```python
from build123d import *

# Parameters (mm, degrees)
SKETCH1_R           = 2.38125
SKETCH1_R_2         = 2.1828125
BOSS_EXTRUDE1_DEPTH = 6.35
CHAMFER1_SIZE       = 3.175
CHAMFER2_SIZE       = 0.396875


with BuildPart() as part:
    # Sketch1 → Boss-Extrude1 (new body)
    with BuildSketch(Plane(origin=(0, 0, 0), x_dir=(1, 0, 0), z_dir=(0, 1, 0))):
        Polygon((-44.45, 6.35), (62.365403734, 6.35), (119.934787808, -51.219384074), (110.954531687, -60.199640195), (57.104891492, -6.35), (-44.45, -6.35), align=None)
        with Locations(Location((-38.1, 0, 0), (0, 0, 270))):
            Circle(SKETCH1_R, mode=Mode.SUBTRACT)
        with Locations(Location((0, 0, 0), (0, 0, 270))):
            Circle(SKETCH1_R, mode=Mode.SUBTRACT)
        with Locations(Location((110.954531687, -51.219384074, 0), (0, 0, 270))):
            Circle(SKETCH1_R_2, mode=Mode.SUBTRACT)
        with Locations(Location((101.974275566, -42.239127953, 0), (0, 0, 270))):
            Circle(SKETCH1_R_2, mode=Mode.SUBTRACT)
        with Locations(Location((-12.7, 0, 0), (0, 0, 270))):
            Circle(SKETCH1_R_2, mode=Mode.SUBTRACT)
        with Locations(Location((25.4, 0, 0), (0, 0, 270))):
            Circle(SKETCH1_R_2, mode=Mode.SUBTRACT)
        with Locations(Location((84.013763324, -24.27861571, 0), (0, 0, 270))):
            Circle(SKETCH1_R_2, mode=Mode.SUBTRACT)
    extrude(amount=BOSS_EXTRUDE1_DEPTH)

    # Fillet1
    # the kernel refuses this chamfer: 50.8 mm, written as the material it adds along each edge
    with BuildSketch(Plane(origin=(57.104891492, 0, 6.35), x_dir=(0.7306772036716535, 0, 0.6827230946984092), z_dir=(0, 1, 0))) as fillet1_piece_1:
        with BuildLine():
            Line((22.93255988, 0), (-17.277556946, -15.079400804))
            Line((-17.277556946, -15.079400804), (-17.97120361, -14.337032765))
            ThreePointArc((-17.97120361, -14.337032765), (-9.066978051, -7.081424312), (-0.693646664, 0.742368039))
            Line((-0.693646664, 0.742368039), (0.034451214, 1.015415734))
            ThreePointArc((0.034451214, 1.015415734), (11.487547245, 0.626832956), (22.967011094, 1.015415734))
            Line((22.967011094, 1.015415734), (22.93255988, 0))
        make_face()
    extrude(amount=6.35)

    # Fillet2
    # the kernel refuses this chamfer: 57.15 mm, written as the material it takes off along each edge
    with BuildSketch(Plane(origin=(62.365403734, -64.497824661, -6.35), x_dir=(0.7306772036716533, 0, 0.6827230946984093), z_dir=(0, 1, 0))) as fillet2_piece_1:
        with BuildLine():
            Line((25.799129864, 0), (-19.437251564, -16.964325904))
            Line((-19.437251564, -16.964325904), (-20.217604061, -16.129161861))
            ThreePointArc((-20.217604061, -16.129161861), (-10.200350307, -7.966602351), (-0.780352497, 0.835164044))
            Line((-0.780352497, 0.835164044), (0.038757616, 1.142342701))
            ThreePointArc((0.038757616, 1.142342701), (12.923490651, 0.705187075), (25.837887481, 1.142342701))
            Line((25.837887481, 1.142342701), (25.799129864, 0))
        make_face()
    extrude(amount=135.345649322, mode=Mode.SUBTRACT)

    # Chamfer1
    chamfer1_edges = [part.edges().sort_by_distance(p)[0] for p in [
        (-44.45, 3.175, -6.35),
        (119.934787808, 3.175, 51.219384074),
        (110.954531687, 3.175, 60.199640195),
        (-44.45, 3.175, 6.35),
    ]]
    chamfer(chamfer1_edges, length=CHAMFER1_SIZE)

    # Chamfer2
    chamfer2_edges = [part.edges().sort_by_distance(p)[0] for p in [
        (0, 0, -2.38125),
        (0, 6.35, -2.38125),
        (-38.1, 0, -2.38125),
        (-38.1, 6.35, -2.38125),
        (110.954531687, 0, 49.036571574),
        (110.954531687, 6.35, 49.036571574),
        (101.974275566, 0, 40.056315453),
        (101.974275566, 6.35, 40.056315453),
        (-12.7, 0, -2.1828125),
        (-12.7, 6.35, -2.1828125),
        (25.4, 0, -2.1828125),
        (25.4, 6.35, -2.1828125),
        (84.013763324, 0, 22.09580321),
        (84.013763324, 6.35, 22.09580321),
        (90.346667332, 0, 39.59177584),
        (90.346667332, 6.35, 39.59177584),
        (54.023354766, 0, 13.789487758),
        (54.023354766, 6.35, 13.789487758),
        (-1.290950678, 0, -6.35),
        (-1.290950678, 6.35, -6.35),
        (58.898674917, 0, 2.019423728),
        (58.898674917, 6.35, 2.019423728),
        (-44.45, 0, 0),
        (-44.45, 6.35, 0),
        (98.396987484, 0, 29.681583749),
        (115.444659748, 0, 55.709512134),
        (-2.606078738, 0, 6.35),
        (117.689723778, 0, 51.219384074),
        (110.954531687, 0, 57.954576164),
        (-42.8625, 0, 4.7625),
        (-42.8625, 0, -4.7625),
        (98.396987484, 6.35, 29.681583749),
        (-2.606078738, 6.35, 6.35),
        (115.444659748, 6.35, 55.709512134),
        (117.689723778, 6.35, 51.219384074),
        (110.954531687, 6.35, 57.954576164),
        (-42.8625, 6.35, 4.7625),
        (-42.8625, 6.35, -4.7625),
    ]]
    chamfer(chamfer2_edges, length=CHAMFER2_SIZE)


solid = part.part
```
Source: CAD feature listing. Evaluate the final solid. Frame: model axes, mm. A direction names the side the tool comes from. Coordinates: 2 decimals unless noted, no trailing zeros. Write each loop counter-clockwise with the first axis right and the second up, starting at its lowest first coordinate (ties: lowest second). Pieces come first, ordered by that corner, then holes. Notation, with made-up numbers: (24.25, 2.25) - (64.25, 2.25) arc R17 cw to (64.25, 15.25) - close; hole circle Ø9 at (1, 37.5). An arc over 180 degrees is marked (long way). Answer as a JSON object with one key per item and string values.
Q1. Material intervals for line 1 (X direction, y = 4.4, z = 0); line 2 (X direction, y = 1.5, z = 49.5); line 3 (Z direction, x = -24, y = 4.25), sorted ascending. Write a range as [from, to].
Ans:
{"line 1": "x = [-44.45, -40.48], [-35.72, -14.88], [-10.52, -2.38], [2.38, 23.22], [27.58, 54.02]", "line 2": "x = [100.25, 109.61], [112.3, 117.69]", "line 3": "z = [-6.35, 6.35]"}
Q2. Section query B-B, the plane y = 2. State how many separate pieces and enclosed holes the cut face has, plus the area to 3 significant figures.
Ans:
{"separate pieces": "1", "enclosed holes": "7", "area": "2,150 mm2"}
Q3. First-contact query: pin 1 Ø3.5 at (x, z) = (84.01, 24.28) entering from -Y; pin 2 Ø1 at (x, y) = (83, 2.5) entering from +Z; pin 3 Ø3 at (x, y) = (-18, 4) entering from +Z; pin 4 Ø2 at (x, y) = (80, 5.5) entering from +Z. Flat tips, straight axial feed; report the tip coordinate or a pass-through.
Ans:
{"pin 1": "passes through", "pin 2": "stops at z = 32.75", "pin 3": "stops at z = 6.35", "pin 4": "stops at z = 30.25"}
Q4. Section query C-C, the plane x = -25. Output: boundary loops of the cut face in (y, z).
Ans:
{"outline": "(0, -5.95) - (0.4, -6.35) - (5.95, -6.35) - (6.35, -5.95) - (6.35, 5.95) - (5.95, 6.35) - (0.4, 6.35) - (0, 5.95) - close"}
Q5. Section query A-A, the plane x = 25.4. Output: boundary loops of the cut face in (y, z).
Ans:
{"outline": "(0, -5.95) - (0.4, -6.35) - (5.95, -6.35) - (6.35, -5.95) - (6.35, -2.58) - (5.95, -2.18) - (0.4, -2.18) - (0, -2.58) - close; (0, 2.58) - (0.4, 2.18) - (5.95, 2.18) - (6.35, 2.58) - (6.35, 5.95) - (5.95, 6.35) - (0.4, 6.35) - (0, 5.95) - close"}
Q6. Draft query along Z for faces 1 (the flat face through (115.334, 6.154, 55.536)), 2 (the cylindrical face through (23.463, 3.136, 1.007)), 3 (the flat face through (97.99, 0.2, 29.55)). Return one class per face: released by +Z, released by -Z, zero draft, split by the parting line, or undercut.
Ans:
{"face 1": "released by +Z", "face 2": "undercut", "face 3": "released by -Z"}
Q7. Set-up query: faces 4 (the flat face through (-2, 3, 6.35)), 5 (the flat face through (-42.7, 0.2, -4.65)). Return all of +Z, -Z, +X, -X, +Y, -Y with unobstructed straight access to the full face (end or side cutting, diameter ignored); none if empty.
Ans:
{"face 4": "+Z, -X, +Y, -Y", "face 5": "-Z, -X, -Y"}
